Answer from the drawing. Dimensions are ordinates in mm from the lowest x, y and z of the part. A direction names the side the tool comes from. Give positions to 0.01 mm unless a question says otherwise; leave off trailing zeros. Loops run counter-clockwise (first coordinate to the right, second up) from the corner with the lowest first, then second, coordinate; pieces in that order, holes last. Notation, with made-up numbers: M -2,-22 L 25,-22 A32 ccw 25,7 Z; hole C 43,-18 d10. An arc over 180 degrees is marked long. Use a Markdown table: item, result.
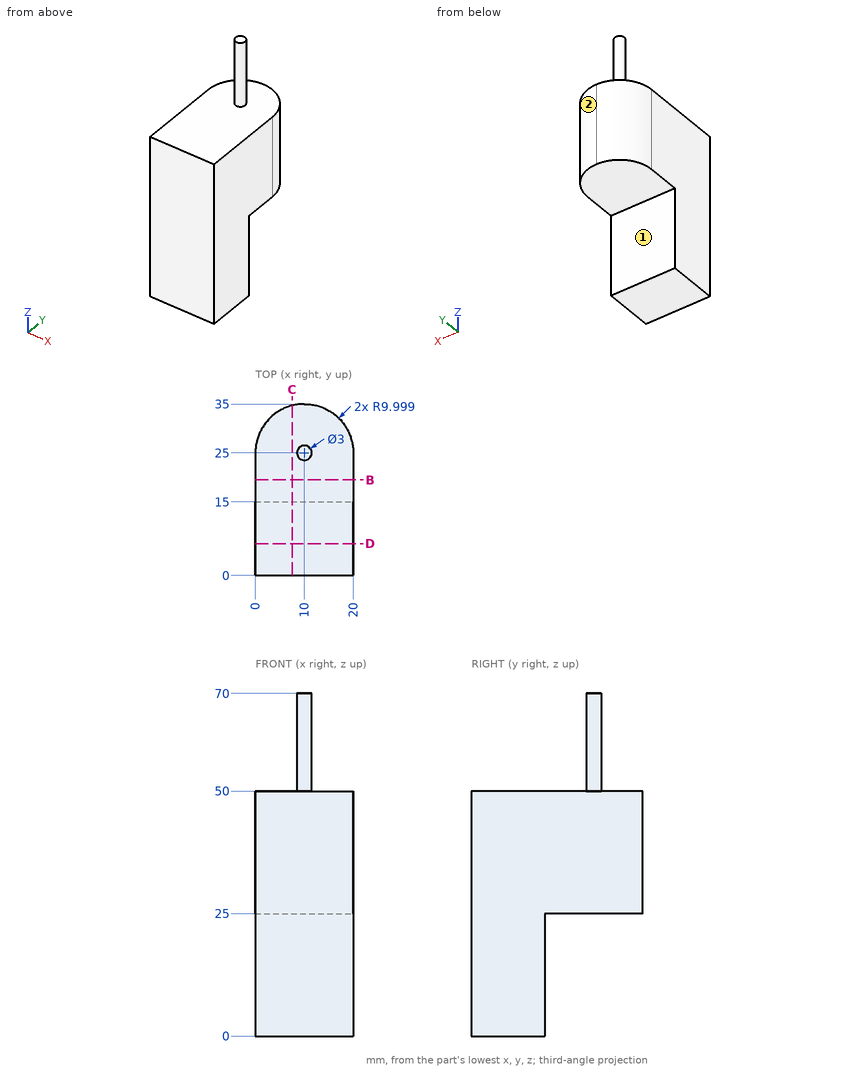
(1) A cutting plane is placed at C-C (x = 7.5). Write down the section's boundary in (y, z), and give its area (3 significant figures).
Entries:
| item | result |
|---|---|
| outline | M 0,0 L 15,0 L 15,25 L 34.68,25 L 34.68,50 L 0,50 Z |
| area | 1,240 mm² |
(2) Consider probe 1 along Z at (x, y) = (8.25, 32); probe 2 along Z at (x, y) = (1.5, 2); probe 3 along Y at (x, z) = (8, 8.5). Determine where each line is inside the solid, lowest interval first. Write a range as [from, to].
Entries:
| item | result |
|---|---|
| probe 1 | z = [25, 50] |
| probe 2 | z = [0, 50] |
| probe 3 | y = [0, 15] |
(3) A cutting plane is placed at D-D (y = 6.5). Write down the section's boundary in (x, z).
Entries:
| item | result |
|---|---|
| outline | M 0,0 L 20,0 L 20,50 L 0,50 Z |
(4) Which of the six approach directions +Z, -Z, +X, -X, +Y, -Y give full straight-line access (tool end or side, diameter ignored) to the marked faces 1 and 2?
Entries:
| item | result |
|---|---|
| face 1 | -Z, +X, -X, +Y |
| face 2 | +Z, -Z, +X, +Y |
(5) Given P1, Ø1.5, axis at x = 13, y = 17.5, coming from the +Z side; P2, Ø12, axis at x = 10.5, z = 61, coming from the -Y side; P3, Ø1.5, axis at x = 14.5, y = 22, coming from the -Z side, each flat-ended and moving along its own axis, determine where each tip first touches the part or whether it passes through.
Entries:
| item | result |
|---|---|
| P1 | stops at z = 50 |
| P2 | stops at y = 23.5 |
| P3 | stops at z = 25 |
(6) A cutting plane is placed at B-B (y = 19.5). Write down the section's boundary in (x, z), and give its area (3 significant figures).
Entries:
| item | result |
|---|---|
| outline | M 0,25 L 20,25 L 20,50 L 0,50 Z |
| area | 500 mm² |
